from build123d import *

# Parameters (mm, degrees)
SKETCH1_R           = 100.33
SKETCH1_R_2         = 86.36
SKETCH1_R_3         = 1.7859375
BOSS_EXTRUDE1_DEPTH = 7.62


with BuildPart() as part:
    # Sketch1 → Boss-Extrude1 (new body)
    with BuildSketch(Plane.XY):
        with Locations(Location((0, 0, 0), (0, 0, 180))):
            Circle(SKETCH1_R)
        with Locations(Location((0, 0, 0), (0, 0, 180))):
            Circle(SKETCH1_R_2, mode=Mode.SUBTRACT)
        with Locations(Location((0, 93.345, 0), (0, 0, 180))):
            Circle(SKETCH1_R_3, mode=Mode.SUBTRACT)
        with Locations(Location((93.345, 0, 0), (0, 0, 180))):
            Circle(SKETCH1_R_3, mode=Mode.SUBTRACT)
        with Locations(Location((0, -93.345, 0), (0, 0, 180))):
            Circle(SKETCH1_R_3, mode=Mode.SUBTRACT)
        with Locations(Location((-93.345, 0, 0), (0, 0, 180))):
            Circle(SKETCH1_R_3, mode=Mode.SUBTRACT)
    extrude(amount=BOSS_EXTRUDE1_DEPTH)


solid = part.part
Verification items for the finished model (mm, model axes). Coordinates: 2 decimals unless noted, no trailing zeros. Loops run counter-clockwise (first coordinate to the right, second up) from the corner with the lowest first, then second, coordinate; pieces in that order, holes last. Notation, with made-up numbers: (21, 66.25) -> (76, 66.25) arc R16 cw to (76, 78.25) -> close; hole circle Ø5 at (25, 71). An arc over 180 degrees is marked (long way). Answer as a JSON object with one key per item and string values. Group by question number.
Item 1: Sectioned sample at B-B on x = 40. Record the boundary of the cut face in (y, z), plus the area to 3 significant figures.
Item 2: Sectioned sample at A-A on y = -42.5. Record the boundary of the cut face in (x, z), plus the area to 3 significant figures.
Item 3: Sectioned sample at C-C on z = 2.5. Record the boundary of the cut face in (x, y) (3 decimals), plus the area to 3 significant figures.
Item 4: Scan lines: probe 1 along Y at (x, z) = (0, 3.5); probe 2 along X at (y, z) = (-3, 4.25); probe 3 along X at (y, z) = (-65, 2). Record each from-to range of solid material in increasing order.
Item 5: Mould release check, pull along Y, two halves, no side actions. Record for faces 1 (the cylindrical face through (63.65, -58.37, 3.76)), 2 (the cylindrical face through (13.061, -99.476, 3.757)), 3 (the flat face through (-44, -75, 7.62)): +Y half, -Y half, draft (parallel to the pull), parting line (faces both ways), or undercut.
Item 6: Depth check by flat-ended pin: pin 1 (2 mm diameter, centred on x = 0, y = -93.345, fed in from +Z); pin 2 (3 mm diameter, centred on x = 62.5, z = 3, fed in from +Y); pin 3 (4 mm diameter, centred on x = -54.5, z = 4.5, fed in from +Y); pin 4 (2 mm diameter, centred on y = 72, z = 4, fed in from -X). Enter the tip coordinate at first touch or a pass-through.
Evaluation:
{
 "1": {"outline": "(-92.01, 0) -> (-76.54, 0) -> (-76.54, 7.62) -> (-92.01, 7.62) -> close; (76.54, 0) -> (92.01, 0) -> (92.01, 7.62) -> (76.54, 7.62) -> close", "area": "236 mm²"},
 "2": {"outline": "(-90.88, 0) -> (-75.18, 0) -> (-75.18, 7.62) -> (-90.88, 7.62) -> close; (75.18, 0) -> (90.88, 0) -> (90.88, 7.62) -> (75.18, 7.62) -> close", "area": "239 mm²"},
 "3": {"outline": "circle Ø200.66 at (0, 0); hole circle Ø3.572 at (-93.345, 0); hole circle Ø172.72 at (0, 0); hole circle Ø3.572 at (0, -93.345); hole circle Ø3.572 at (0, 93.345); hole circle Ø3.572 at (93.345, 0)", "area": "8,150 mm²"},
 "4": {"probe 1": "y = -100.33 to -95.13, -91.56 to -86.36, 86.36 to 91.56, 95.13 to 100.33", "probe 2": "x = -100.29 to -86.31, 86.31 to 100.29", "probe 3": "x = -76.43 to -56.86, 56.86 to 76.43"},
 "5": {"face 1": "undercut", "face 2": "parting line", "face 3": "draft"},
 "6": {"pin 1": "passes through", "pin 2": "stops at y = 79.66", "pin 3": "stops at y = 85.5", "pin 4": "stops at x = -70.89"}
}
